Part model, mm, in its own coordinate system. A direction names the side the tool comes from. Round coordinates to 2 decimals unless told otherwise and drop trailing zeros. Write each loop counter-clockwise with the first axis right and the second up, starting at its lowest first coordinate (ties: lowest second). Pieces come first, ordered by that corner, then holes.
1) Which spindle directions (+Z, -Z, +X, -X, +Y, -Y) get a long thin tool onto all of the face, cutting with end or side? Do faces 1 (the flat face through (20, -33, 12)), 2 (the flat face through (32, -46, 7.25)), 3 (the cylindrical face through (31.466, -2.465, 18.979)). Say none if no direction does.
2) Saw through at C-C on z = 13. Write the cut outline in (x, y).
3) Saw through at A-A on z = 5.5. Write the cut outline in (x, y).
4) Pull direction X, two halves, no side cores. Call faces 4 (the cylindrical face through (27.599, -27.185, 3.252)), 5 (the flat face through (0, -8, 12)), 6 (the flat face through (28, -50, 3)): +X half, -X half, draft (parallel to the pull), parting line (faces both ways), or undercut.
5) Saw through at B-B on y = -13. Write the cut outline in (x, z), and give its area (3 significant figures).
6) Flat gauge pins, fed straight in: pin 1 (4 mm diameter, centred on x = 26.5, z = 6, fed in from +Y); pin 2 (2 mm diameter, centred on y = -37, z = 15.5, fed in from -X). Where does each tip first touch, or does it go through?
7) Drill centre lines: L1, parallel to X at y = -3, z = 5.5; L2, parallel to Z at x = 27.5, y = -21; L3, parallel to Z at x = 25, y = -47. Where is each one in solid material? Low to high.
8) Saw through at D-D on x = 8. Write the cut outline in (y, z), and give its area (3 significant figures).
```python
from build123d import *

# Parameters (mm, degrees)
EXTRUDE_1_DEPTH     = 25
SKETCH_2_R          = 2.25
CUT_EXTRUDE_1_DEPTH = 66.954529791
SKETCH_3_R          = 4
CUT_EXTRUDE_2_DEPTH = 5
SKETCH_4_W          = 10.5
SKETCH_4_H          = 16
CUT_EXTRUDE_5_DEPTH = 66.954529791


with BuildPart() as part:
    # 草图1 → 凸台-拉伸1 (new body)
    with BuildSketch(Plane.XY):
        Polygon((0, 0), (35, 0), (35, -50), (20, -50), (20, -15), (0, -15), align=None)
    extrude(amount=EXTRUDE_1_DEPTH)

    # 草图2 → 切除-拉伸1 (cut, through all)
    with BuildSketch(Plane(origin=(0, 0, 0), x_dir=(1, 0, 0), z_dir=(0, 1, 0))):
        with Locations(Location((27.5, -5.5, 0), (0, 0, 270))):
            Circle(SKETCH_2_R)
        with Locations(Location((27.5, -19.5, 0), (0, 0, 270))):
            Circle(SKETCH_2_R)
    extrude(amount=-CUT_EXTRUDE_1_DEPTH, mode=Mode.SUBTRACT)

    # 草图3 → 切除-拉伸2 (cut)
    with BuildSketch(Plane(origin=(0, 0, 0), x_dir=(1, 0, 0), z_dir=(0, 1, 0))):
        with Locations(Location((27.5, -5.5, 0), (0, 0, 270))):
            Circle(SKETCH_3_R)
        with Locations(Location((27.5, -19.5, 0), (0, 0, 270))):
            Circle(SKETCH_3_R)
    extrude(amount=-CUT_EXTRUDE_2_DEPTH, mode=Mode.SUBTRACT)

    # 草图4 → 切除-拉伸5 (cut, through all)
    with BuildSketch(Plane(origin=(35, 0, 0), x_dir=(0, 0, -1), z_dir=(1, 0, 0))):
        with Locations((-12.5, -50)):
            Rectangle(SKETCH_4_W, SKETCH_4_H)
    extrude(amount=-CUT_EXTRUDE_5_DEPTH, mode=Mode.SUBTRACT)


solid = part.part
```
Completed:
1. face 1: +Z, -Z, -X, -Y
1. face 2: +X, -X, -Y
1. face 3: +Y
2. outline: (0, -15) - (20, -15) - (20, -42) - (35, -42) - (35, 0) - (0, 0) - close
3. outline: (0, -15) - (20, -15) - (20, -50) - (25.25, -50) - (25.25, -5) - (23.5, -5) - (23.5, 0) - (0, 0) - close; (29.75, -50) - (35, -50) - (35, 0) - (31.5, 0) - (31.5, -5) - (29.75, -5) - close
4. face 4: undercut
4. face 5: -X half
4. face 6: draft
5. outline: (0, 0) - (35, 0) - (35, 25) - (0, 25) - close; hole circle Ø4.5 at (27.5, 5.5); hole circle Ø4.5 at (27.5, 19.5)
5. area: 843 mm2
6. pin 1: stops at y = -5
6. pin 2: stops at x = 20
7. L1: x = 0 to 23.5, 31.5 to 35
7. L2: z = 0 to 3.25, 7.75 to 17.25, 21.75 to 25
7. L3: z = 0 to 7.25, 17.75 to 25
8. outline: (-15, 0) - (0, 0) - (0, 25) - (-15, 25) - close
8. area: 375 mm2
